The model under review builds one solid part; all positions refer to its coordinate system, in mm. Face numbers are marked on the shaded views. A direction names the side the tool comes from. Coordinates: 2 decimals unless noted, no trailing zeros. Order: outer loops, then holes, each group sorted by start corner. A loop starts at its lowest first (then second) coordinate and runs counter-clockwise, first axis right, second up. Notation, with made-up numbers: (14, -32.5) -> (43, -32.5) arc R24 ccw to (43, 0.5) -> close; hole circle Ø8 at (3.25, -32.5). An arc over 180 degrees is marked (long way). Use one line per item in the form item = value.
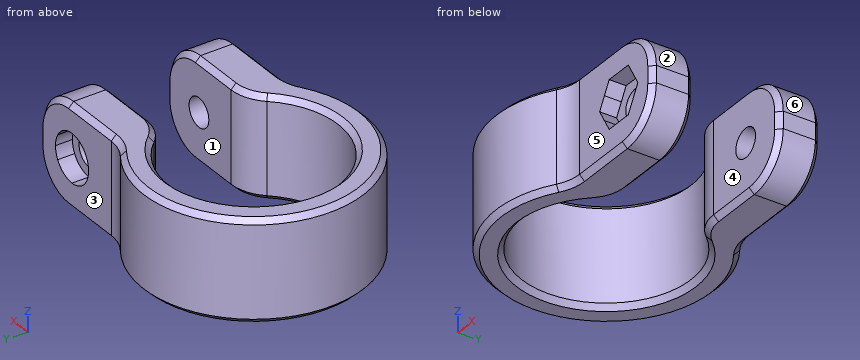
from build123d import *

# Parameters (mm, degrees)
F1_DEPTH = 12
F2_R     = 5
F3_R     = 5
F4_SIZE  = 0.6
F5_R     = 1.7
F6_DEPTH = 23.001
F7_DEPTH = 2
F8_START = -18
F8_DEPTH = 2


with BuildPart() as f1:
    # F0 (on Top) → F1 (new body)
    with BuildSketch(Plane.XY):
        with BuildLine():
            ThreePointArc((8.3066238629, 5.5677643628), (8.4881874106, 5.2868397443), (8.6602540378, 5))
            Line((8.6602540378, 5), (12, 5))
            ThreePointArc((12, 5), (10.4565645973, 7.7240052319), (8.3066238629, 10))
            Line((8.3066238629, 10), (8.3066238629, 5.5677643628))
        make_face()
        with BuildLine():
            ThreePointArc((8.3066238629, 10), (10.4565645973, 7.7240052319), (12, 5))
            Line((12, 5), (22.3066238629, 5))
            Line((22.3066238629, 5), (22.3066238629, 10))
            Line((22.3066238629, 10), (8.3066238629, 10))
        make_face()
        with BuildLine():
            Line((22.3066238629, -5), (12, -5))
            ThreePointArc((12, -5), (10.4565645973, -7.7240052319), (8.3066238629, -10))
            Line((8.3066238629, -10), (22.3066238629, -10))
            Line((22.3066238629, -10), (22.3066238629, -5))
        make_face()
        with BuildLine():
            ThreePointArc((8.3066238629, -5.5677643628), (-10, 0), (8.3066238629, 5.5677643628))
            Line((8.3066238629, 5.5677643628), (8.3066238629, 10))
            ThreePointArc((8.3066238629, 10), (-13, 0), (8.3066238629, -10))
            Line((8.3066238629, -10), (8.3066238629, -5.5677643628))
        make_face()
        with BuildLine():
            Line((12, -5), (8.6602540378, -5))
            ThreePointArc((8.6602540378, -5), (8.4881874106, -5.2868397443), (8.3066238629, -5.5677643628))
            Line((8.3066238629, -5.5677643628), (8.3066238629, -10))
            ThreePointArc((8.3066238629, -10), (10.4565645973, -7.7240052319), (12, -5))
        make_face()
    extrude(amount=F1_DEPTH)

    # F2
    f2_edges = [f1.edges().sort_by_distance(p)[0] for p in [
        (8.306624, -10, 6),
        (8.306624, 10, 6),
        (8.660254, -5, 6),
        (8.660254, 5, 6),
    ]]
    fillet(f2_edges, radius=F2_R)

    # F3
    f3_edges = [f1.edges().sort_by_distance(p)[0] for p in [
        (22.306624, -7.5, 12),
        (22.306624, 7.5, 12),
        (22.306624, -7.5, 0),
        (22.306624, 7.5, 0),
    ]]
    fillet(f3_edges, radius=F3_R)

    # F4
    f4_edges = [f1.edges().sort_by_distance(p)[0] for p in [
        (-10, 0, 12),
        (-13, 0, 12),
        (-13, 0, 0),
        (-10, 0, 0),
    ]]
    chamfer(f4_edges, length=F4_SIZE)

    # F5 (on face) → F6 (cut, through all)
    with BuildSketch(Plane.XZ.offset(10)):
        with Locations((16.7066238629, 6)):
            Circle(F5_R)
    extrude(amount=-F6_DEPTH, mode=Mode.SUBTRACT)

    # F5 (on face) → F7 (cut)
    with BuildSketch(Plane.XZ.offset(10)):
        with BuildLine():
            ThreePointArc((19.1747962235, 4.5749999304), (19.4595124574, 5.2623656827), (19.5566238629, 6))
            ThreePointArc((19.5566238629, 6), (19.4595124887, 6.7376342007), (19.1747963443, 7.4249998605))
            ThreePointArc((19.1747963443, 7.4249998605), (18.1316239327, 8.4681723605), (16.7066238629, 8.85))
            ThreePointArc((16.7066238629, 8.85), (15.2816238977, 8.4681724209), (14.2384515023, 7.4250000696))
            ThreePointArc((14.2384515023, 7.4250000696), (13.8566238629, 6.0000000373), (14.238451465, 4.574999995))
            ThreePointArc((14.238451465, 4.574999995), (15.2816238654, 3.5318275978), (16.7066238629, 3.15))
            ThreePointArc((16.7066238629, 3.15), (18.1316238281, 3.5318275791), (19.1747962235, 4.5749999304))
        make_face()
        with Locations((16.7066238629, 6)):
            Circle(F5_R, mode=Mode.SUBTRACT)
        with BuildLine():
            Line((15.0611755957, 3.15), (16.7066238629, 3.15))
            ThreePointArc((16.7066238629, 3.15), (15.2816238654, 3.5318275978), (14.238451465, 4.574999995))
            Line((14.238451465, 4.574999995), (15.0611755957, 3.15))
        make_face()
        with BuildLine():
            Line((18.3520721301, 3.15), (19.1747962235, 4.5749999304))
            ThreePointArc((19.1747962235, 4.5749999304), (18.1316238281, 3.5318275791), (16.7066238629, 3.15))
            Line((16.7066238629, 3.15), (18.3520721301, 3.15))
        make_face()
        with BuildLine():
            ThreePointArc((19.1747963443, 7.4249998605), (19.4595124887, 6.7376342007), (19.5566238629, 6))
            ThreePointArc((19.5566238629, 6), (19.4595124574, 5.2623656827), (19.1747962235, 4.5749999304))
            Line((19.1747962235, 4.5749999304), (19.9975203973, 6))
            Line((19.9975203973, 6), (19.1747963443, 7.4249998605))
        make_face()
        with BuildLine():
            ThreePointArc((16.7066238629, 8.85), (18.1316239327, 8.4681723605), (19.1747963443, 7.4249998605))
            Line((19.1747963443, 7.4249998605), (18.3520721301, 8.85))
            Line((18.3520721301, 8.85), (16.7066238629, 8.85))
        make_face()
        with BuildLine():
            ThreePointArc((14.238451465, 4.574999995), (13.8566238629, 6.0000000373), (14.2384515023, 7.4250000696))
            Line((14.2384515023, 7.4250000696), (13.4157273285, 6))
            Line((13.4157273285, 6), (14.238451465, 4.574999995))
        make_face()
        with BuildLine():
            ThreePointArc((14.2384515023, 7.4250000696), (15.2816238977, 8.4681724209), (16.7066238629, 8.85))
            Line((16.7066238629, 8.85), (15.0611755957, 8.85))
            Line((15.0611755957, 8.85), (14.2384515023, 7.4250000696))
        make_face()
    extrude(amount=-F7_DEPTH, mode=Mode.SUBTRACT)

    # F5 (on face) → F8 (cut)
    with BuildSketch(Plane.XZ.offset(10).offset(F8_START)):
        with BuildLine():
            ThreePointArc((19.1747962235, 4.5749999304), (19.4595124574, 5.2623656827), (19.5566238629, 6))
            ThreePointArc((19.5566238629, 6), (19.4595124887, 6.7376342007), (19.1747963443, 7.4249998605))
            ThreePointArc((19.1747963443, 7.4249998605), (18.1316239327, 8.4681723605), (16.7066238629, 8.85))
            ThreePointArc((16.7066238629, 8.85), (15.2816238977, 8.4681724209), (14.2384515023, 7.4250000696))
            ThreePointArc((14.2384515023, 7.4250000696), (13.8566238629, 6.0000000373), (14.238451465, 4.574999995))
            ThreePointArc((14.238451465, 4.574999995), (15.2816238654, 3.5318275978), (16.7066238629, 3.15))
            ThreePointArc((16.7066238629, 3.15), (18.1316238281, 3.5318275791), (19.1747962235, 4.5749999304))
        make_face()
        with Locations((16.7066238629, 6)):
            Circle(F5_R, mode=Mode.SUBTRACT)
    extrude(amount=-F8_DEPTH, mode=Mode.SUBTRACT)


solid = f1.part
Item 1: We need section B-B (y = 0). Write out the cut boundary in (x, z), plus the area to 3 significant figures.
Results found:
outline = (-13, 0.6) -> (-12.4, 0) -> (-10.6, 0) -> (-10, 0.6) -> (-10, 11.4) -> (-10.6, 12) -> (-12.4, 12) -> (-13, 11.4) -> close
area = 35.3 mm²
Item 2: To check wall thickness, follow L1, parallel to Y at x = 20, z = 2.25; L2, parallel to Y at x = 15, z = 6.5; L3, parallel to X at y = 0, z = 7. State the ranges of each line that lie inside material, in increasing order. Write a range as from..to.
Results found:
L1 = -10..-5, 5..10
L2 = -8..-5, 5..8
L3 = -13..-10
Item 3: We need section A-A (x = 15.5). State how many separate pieces and enclosed holes the cut face has, plus the area to 3 significant figures.
Results found:
separate_pieces = 4
enclosed_holes = 0
area = 82.5 mm²
Item 4: Tool access review of the marked faces 1 and 2: name each direction out of +Z, -Z, +X, -X, +Y, -Y from which nothing blocks a thin tool from reaching the whole face with its end or side.
Results found:
face_1 = +Z, -Z, +X
face_2 = +Z, +X, +Y, -Y
Item 5: Clearance check with flat-ended pins moving along their axes: pin 1 (2 mm diameter, centred on x = 16, y = -9.5, fed in from +Z); pin 2 (4 mm diameter, centred on y = -2, z = 11, fed in from +X); pin 3 (3 mm diameter, centred on x = 9, y = -2, fed in from +Z); pin 4 (4.5 mm diameter, centred on x = 16.5, z = 5.5, fed in from -Y). State where each tip first meets the part, or that it passes through.
Results found:
pin_1 = 12
pin_2 = -9.17
pin_3 = through
pin_4 = -8
Item 6: Draft analysis for pull direction Y (two halves, no side actions). For the marked faces 3, 4, 5 and 6, state which applies: released by +Y, released by -Y, zero draft, split by the parting line, or undercut.
Results found:
face_3 = released by +Y
face_4 = undercut
face_5 = released by -Y
face_6 = zero draft
